Design review of the part built by this model. Coordinates are the model's own, in mm. A direction names the side the tool comes from. Round coordinates to 2 decimals unless told otherwise and drop trailing zeros. Loops run counter-clockwise (first coordinate to the right, second up) from the corner with the lowest first, then second, coordinate; pieces in that order, holes last. Notation, with made-up numbers: (73, -40) - (118, -40) arc R21 cw to (118, -19) - close; hole circle Ø5 at (81.5, 4.5). An arc over 180 degrees is marked (long way). Use one line per item in the form item = value. Start each with the question number.
(1) Wall thickness on probe 1 along Y at (x, z) = (-12, -6.5); probe 2 along X at (y, z) = (1.25, -5.25); probe 3 along Z at (x, y) = (-4, 8): over which ranges is each line inside the solid? List them lowest first. Write a range as [from, to].
(2) For pin 1 (0.9 mm diameter, centred on x = -26.5, y = 5.5, fed in from +Z), flat-tipped, find the tip position at first contact; note if it passes through.
(3) Machinability: for faces 4 (the flat face through (0, 5, -10)), 5 (the cylindrical face through (-10.77, 6.44, -4.93)), which of the approach directions +Z, -Z, +X, -X, +Y, -Y give a long, thin tool a straight path to every point of the face, cutting with its end or side? Answer none if there is none.
(4) The part is to be moulded in two halves that separate along Z. For faces 1 (the flat face through (-19, 5, -20.828)), 2 (the cylindrical face through (-8.51, 4.93, -8.21)), 3 (the flat face through (-19, 10, -11)), say which applies: released by +Z, released by -Z, zero draft, split by the parting line, or undercut.
(5) We need section D-D, the plane x = -12. Write out the cut boundary in (y, z), then the cut area to 3 significant figures.
(6) We need section B-B, the plane z = -7.5. Write out the cut boundary in (x, y).
(7) We need section A-A, the plane x = -6.35. Write out the cut boundary in (y, z).
(8) We need section C-C, the plane y = 6. Write out the cut boundary in (x, z), then the cut area to 3 significant figures.
from build123d import *

# Parameters (mm, degrees)
SKETCH1_W           = 38.1
SKETCH1_H           = 20.828
SKETCH1_R           = 2.564
BOSS_EXTRUDE1_DEPTH = 10
SKETCH2_R           = 1.55
CUT_EXTRUDE1_DEPTH  = 10


with BuildPart() as part:
    # Sketch1 → Boss-Extrude1 (new body)
    with BuildSketch(Plane(origin=(0, 0, 0), x_dir=(1, 0, 0), z_dir=(0, 1, 0))):
        with Locations((-19.05, 10.414)):
            Rectangle(SKETCH1_W, SKETCH1_H)
        with Locations(Location((-31.75, 6.828, 0), (0, 0, 270))):
            Circle(SKETCH1_R, mode=Mode.SUBTRACT)
        with Locations(Location((-6.35, 6.828, 0), (0, 0, 90))):
            Circle(SKETCH1_R, mode=Mode.SUBTRACT)
    extrude(amount=BOSS_EXTRUDE1_DEPTH)

    # Sketch2 → Cut-Extrude1 (cut)
    with BuildSketch(Plane.XY):
        with Locations((-26.1, 5.5)):
            Circle(SKETCH2_R)
        with Locations(Location((-12, 5.5, 0), (0, 0, 180))):
            Circle(SKETCH2_R)
    extrude(amount=-CUT_EXTRUDE1_DEPTH, mode=Mode.SUBTRACT)


solid = part.part
Data:
q1.probe_1 = [0, 3.95], [7.05, 10]
q1.probe_2 = [-38.1, -33.77], [-29.73, -8.37], [-4.33, 0]
q1.probe_3 = [-20.83, -7.85], [-5.8, 0]
q2.pin_1 = -10
q3.face_4 = +Z, -Z, +X, +Y, -Y
q3.face_5 = +Z
q4.face_1 = released by -Z
q4.face_2 = undercut
q4.face_3 = zero draft
q5.outline = (0, -20.83) - (10, -20.83) - (10, 0) - (7.05, 0) - (7.05, -10) - (3.95, -10) - (3.95, 0) - (0, 0) - close
q5.area = 177 mm^2
q6.outline = (-38.1, 0) - (-34.22, 0) - (-34.22, 10) - (-38.1, 10) - close; (-29.28, 0) - (-8.82, 0) - (-8.82, 10) - (-29.28, 10) - close; (-3.88, 0) - (0, 0) - (0, 10) - (-3.88, 10) - close; hole circle Ø3.1 at (-26.1, 5.5); hole circle Ø3.1 at (-12, 5.5)
q7.outline = (0, -20.83) - (10, -20.83) - (10, -9.39) - (0, -9.39) - close; (0, -4.26) - (10, -4.26) - (10, 0) - (0, 0) - close
q8.outline = (-38.1, -20.83) - (0, -20.83) - (0, 0) - (-10.53, 0) - (-10.53, -10) - (-13.47, -10) - (-13.47, 0) - (-24.63, 0) - (-24.63, -10) - (-27.57, -10) - (-27.57, 0) - (-38.1, 0) - close; hole circle Ø5.13 at (-31.75, -6.83); hole circle Ø5.13 at (-6.35, -6.83)
q8.area = 694 mm^2
